Check sheet for the modelled part. Datum: model origin and axes. Units: mm. Coordinates: 2 decimals unless noted, no trailing zeros. Order: outer loops, then holes, each group sorted by start corner. A loop starts at its lowest first (then second) coordinate and runs counter-clockwise, first axis right, second up.
Autodesk Inventor part; units mm, degrees
ref_plane "YZ Plane" through (0, 0, 0) normal (1, 0, 0) x (0, 1, 0)
ref_plane "XZ Plane" through (0, 0, 0) normal (0, 1, 0) x (-1, 0, 0)
ref_plane "XY Plane" through (0, 0, 0) normal (0, 0, 1) x (1, 0, 0)
sketch "Sketch1" plane through (0, 0, 0) normal (0, 1, 0) x (-1, 0, 0)
  line L0 (20, 10) -> (0, 10)
  line L1 (0, 10) -> (20, 10)
  line L2 (20, 10) -> (20, 0)
  line L3 (20, 0) -> (0, 0)
  line L4 (0, 0) -> (0, 10)
  line L5 (0, 10) -> (2.5, 10)
  circle A0 centre (2.5, 8.5) radius 0.5
  circle A1 centre (2.5, 1.5) radius 0.5
  circle A2 centre (17.5, 1.5) radius 0.5
  circle A3 centre (17.5, 8.5) radius 0.5
  point P0 (0, 0)
  point P1 (10, 0)
  point P2 (10, 0)
  point P3 (16.8377, 0)
  point P4 (20, 10)
  dimension "d0" = 20
  dimension "d1" = 2.5
  dimension "d2" = 1
  dimension "d3" = 1
  dimension "d4" = 1
  dimension "d5" = 1
extrude "Extrusion1" add sketch "Sketch1" along normal blind 2
properties part number "bracket"
(1) Cross-section at A-A (z = 1.5). Enter the section's corners in (x, y), and give its area (3 significant figures).
Filled in:
outline: (-20, 0) - (-18, 0) - (-18, 2) - (-20, 2) - close; (-17, 0) - (-3, 0) - (-3, 2) - (-17, 2) - close; (-2, 0) - (0, 0) - (0, 2) - (-2, 2) - close
area: 36.0 mm2
(2) Release check for a two-part mould opening along Z. For faces 1 (the flat face through (-10, 0, 5)), 2 (the cylindrical face through (-17.731, 0.986, 8.944)), 3 (the flat face through (-10, 1, 0)), 4 (the flat face through (-10, 1, 10)) record: +Z half, -Z half, draft (parallel to the pull), parting line (faces both ways), or undercut.
Filled in:
face 1: draft
face 2: undercut
face 3: -Z half
face 4: +Z half
(3) Cross-section at B-B (x = -17.5). Enter the section's corners in (y, z).
Filled in:
outline: (0, 0) - (2, 0) - (2, 1) - (0, 1) - close; (0, 2) - (2, 2) - (2, 8) - (0, 8) - close; (0, 9) - (2, 9) - (2, 10) - (0, 10) - close
(4) Cross-section at C-C (y = 1.8). Enter the section's corners in (x, z).
Filled in:
outline: (-20, 0) - (0, 0) - (0, 10) - (-20, 10) - close; hole circle Ø1 at (-17.5, 1.5); hole circle Ø1 at (-17.5, 8.5); hole circle Ø1 at (-2.5, 1.5); hole circle Ø1 at (-2.5, 8.5)
(5) Thickness scan on probe 1 along Z at (x, y) = (-17.5, 1.2); probe 2 along Z at (x, y) = (-17.75, 0.25). Record the ranges inside material, lowest first.
Filled in:
probe 1: z = 0 to 1, 2 to 8, 9 to 10
probe 2: z = 0 to 1.07, 1.93 to 8.07, 8.93 to 10
